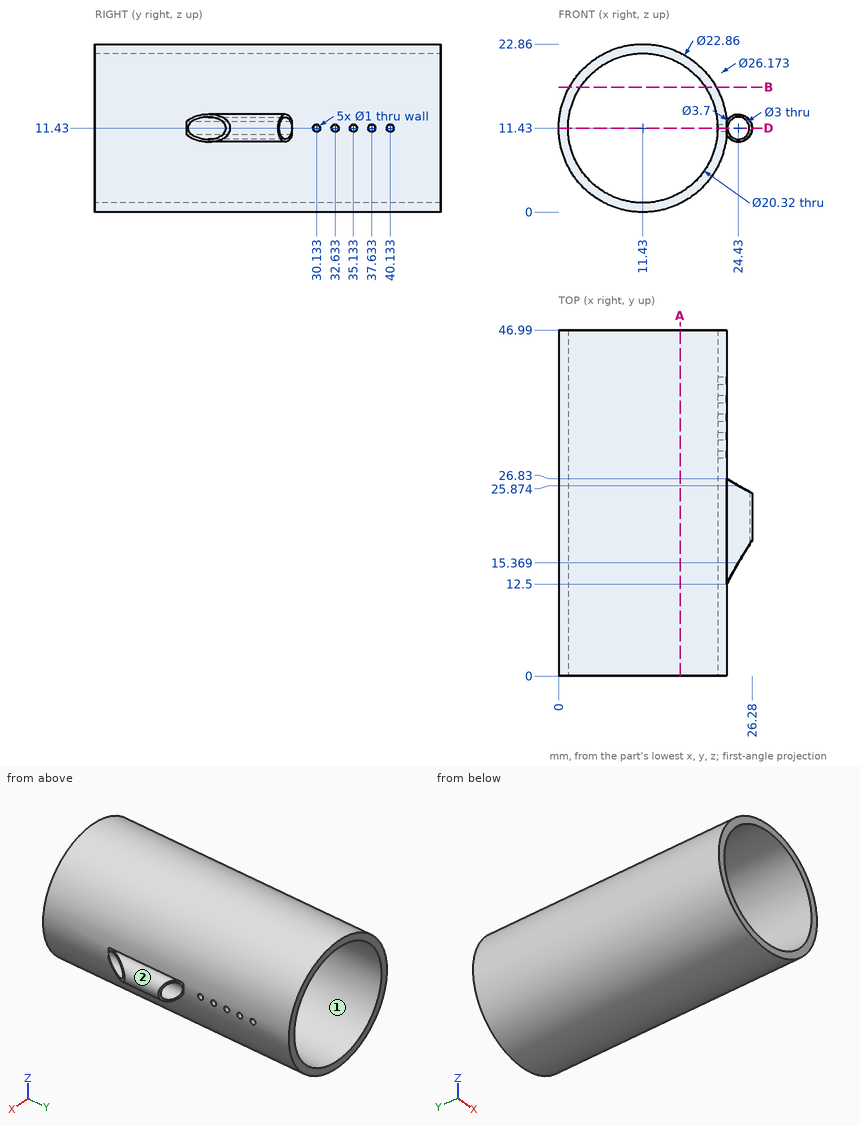
Answer from the drawing. Dimensions are ordinates in mm from the lowest x, y and z of the part. Round coordinates to 2 decimals unless told otherwise and drop trailing zeros. Loops run counter-clockwise (first coordinate to the right, second up) from the corner with the lowest first, then second, coordinate; pieces in that order, holes last.
1) A cutting plane is placed at A-A on x = 16.5. Determine the outline of the cut face in (y, z) (1 decimal).
Outcome:
outline: (0, 1.2) - (47, 1.2) - (47, 2.6) - (0, 2.6) - close; (0, 20.2) - (47, 20.2) - (47, 21.7) - (0, 21.7) - close
2) Consider line 1 (Y direction, x = 21.9, z = 11.43); line 2 (X direction, y = 21.5, z = 11.43); line 3 (Z direction, x = 9, y = 40) (1 decimal). Determine where each line is inside the solid, lowest interval first.
Outcome:
line 1: y = 0 to 29.63, 30.63 to 32.13, 33.13 to 34.63, 35.63 to 37.13, 38.13 to 39.63, 40.63 to 46.99
line 2: x = 0 to 1.27, 21.59 to 22.93, 25.93 to 26.28
line 3: z = 0.3 to 1.6, 21.3 to 22.6
3) A cutting plane is placed at B-B on z = 17. Determine the outline of the cut face in (x, y).
Outcome:
outline: (1.45, 0) - (2.93, 0) - (2.93, 46.99) - (1.45, 46.99) - close; (19.93, 0) - (21.41, 0) - (21.41, 46.99) - (19.93, 46.99) - close
4) For a pull along X with two mould halves and no side action, classify the marked faces 1 and 2 as released by +X, released by -X, zero draft, split by the parting line, or undercut.
Outcome:
face 1: undercut
face 2: undercut
5) A cutting plane is placed at D-D on z = 11.43. Give the number of separate pieces and of enclosed holes in the cut face.
Outcome:
separate pieces: 8
enclosed holes: 0
6) Given P1, Ø2.5, axis at x = 24.43, z = 11.43, coming from the +Y side; P2, Ø1, axis at y = 42, z = 6.5, coming from the -X side; P3, Ø1.5, axis at y = 16.5, z = 6.5, coming from the +X side; P4, Ø12, axis at y = 22.5, z = 7, coming from the +X side, each flat-ended and moving along its own axis, determine where each tip first touches the part or whether it passes through.
Outcome:
P1: passes through
P2: stops at x = 0.89
P3: stops at x = 22.07
P4: stops at x = 26.28
